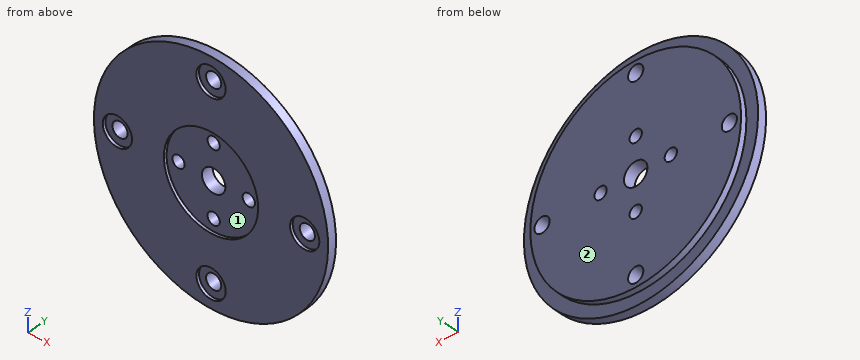
```python
from build123d import *

# Parameters (mm, degrees)
SKETCH_1_R               = 40
EXTRUDE_1_DEPTH          = 3
SKETCH_2_R               = 36
EXTRUDE_2_DEPTH          = 2
CUT_EXTRUDE_1_DEPTH      = 57.789083458
CUT_EXTRUDE_1_DEPTH_BACK = 57.789083458
SKETCH_3_R               = 2.1
SKETCH_3_R_2             = 4
SKETCH_4_R               = 16.1
CUT_EXTRUDE_2_DEPTH      = 1
SKETCH_5_R               = 2.6
CUT_EXTRUDE_3_DEPTH      = 57.789083458
SKETCH_6_R               = 5
CUT_EXTRUDE_4_DEPTH      = 1


with BuildPart() as part:
    # 草图1 → 凸台-拉伸1 (new body)
    with BuildSketch(Plane(origin=(0, 0, 0), x_dir=(1, 0, 0), z_dir=(0, 1, 0))):
        with Locations(Location((0, 0, 0), (0, 0, 270))):
            Circle(SKETCH_1_R)
    extrude(amount=EXTRUDE_1_DEPTH)

    # 草图2 → 凸台-拉伸2 (add)
    with BuildSketch(Plane(origin=(0, 3, 0), x_dir=(1, 0, 0), z_dir=(0, 1, 0))):
        with Locations(Location((0, 0, 0), (0, 0, 270))):
            Circle(SKETCH_2_R)
    extrude(amount=EXTRUDE_2_DEPTH)

    # 草图3 → 切除-拉伸1 (cut, two sides: drawn at the far end of the back side and taken through both)
    with BuildSketch(Plane.XZ.offset(-CUT_EXTRUDE_1_DEPTH_BACK)):
        with Locations(Location((-12, 0, 0), (0, 0, 270))):
            Circle(SKETCH_3_R)
        with Locations(Location((0, 12, 0), (0, 0, 270))):
            Circle(SKETCH_3_R)
        with Locations(Location((12, 0, 0), (0, 0, 270))):
            Circle(SKETCH_3_R)
        with Locations(Location((0, -12, 0), (0, 0, 270))):
            Circle(SKETCH_3_R)
        with Locations(Location((0, 0, 0), (0, 0, 270))):
            Circle(SKETCH_3_R_2)
    extrude(amount=CUT_EXTRUDE_1_DEPTH + CUT_EXTRUDE_1_DEPTH_BACK, mode=Mode.SUBTRACT)

    # 草图4 → 切除-拉伸2 (cut)
    with BuildSketch(Plane.XZ):
        with Locations(Location((0, 0, 0), (0, 0, 270))):
            Circle(SKETCH_4_R)
    extrude(amount=-CUT_EXTRUDE_2_DEPTH, mode=Mode.SUBTRACT)

    # 草图5 → 切除-拉伸3 (cut, through all)
    with BuildSketch(Plane.XZ):
        with Locations(Location((-32, 0, 0), (0, 0, 270))):
            Circle(SKETCH_5_R)
        with Locations(Location((0, 32, 0), (0, 0, 270))):
            Circle(SKETCH_5_R)
        with Locations(Location((32, 0, 0), (0, 0, 270))):
            Circle(SKETCH_5_R)
        with Locations(Location((0, -32, 0), (0, 0, 270))):
            Circle(SKETCH_5_R)
    extrude(amount=-CUT_EXTRUDE_3_DEPTH, mode=Mode.SUBTRACT)

    # 草图6 → 切除-拉伸4 (cut)
    with BuildSketch(Plane.XZ):
        with Locations(Location((0, -32, 0), (0, 0, 270))):
            Circle(SKETCH_6_R)
        with Locations(Location((32, 0, 0), (0, 0, 270))):
            Circle(SKETCH_6_R)
        with Locations(Location((0, 32, 0), (0, 0, 270))):
            Circle(SKETCH_6_R)
        with Locations(Location((-32, 0, 0), (0, 0, 270))):
            Circle(SKETCH_6_R)
    extrude(amount=-CUT_EXTRUDE_4_DEPTH, mode=Mode.SUBTRACT)


solid = part.part
```
Could you check a few things on this model? Use its own coordinates, in mm. Face numbers are marked on the shaded views. Round coordinates to 2 decimals unless told otherwise and drop trailing zeros. Loops run counter-clockwise (first coordinate to the right, second up) from the corner with the lowest first, then second, coordinate; pieces in that order, holes last. Notation, with made-up numbers: (29, -34.75) -> (55, -34.75) arc R24 ccw to (55, -21.75) -> close; hole circle Ø10 at (81, 68). An arc over 180 degrees is marked (long way). One line per question, with ' | ' between items.
(1) If we section it at A-A on y = 3.8: Count the separate pieces of the cut face and the enclosed holes in it, and give its area (3 significant figures).
Model answer:
separate pieces: 1 | enclosed holes: 9 | area: 3,880 mm^2
(2) For pin 1 Ø5 at (x, z) = (0, -30.5) entering from -Y; pin 2 Ø3 at (x, y) = (-8.5, 2) entering from +Z; pin 3 Ø2 at (y, z) = (2, -2.5) entering from -X, each with a flat end and sliding along its axis, tell me the tip position at first contact or that it passes through.
Model answer:
pin 1: stops at y = 1 | pin 2: stops at z = 39.38 | pin 3: stops at x = -39.97
(3) If we section it at C-C on x = -32: List the corners of the cut face in (y, z) for me.
Model answer:
outline: (0, -24) -> (3, -24) -> (3, -16.49) -> (5, -16.49) -> (5, -2.6) -> (1, -2.6) -> (1, -5) -> (0, -5) -> close; (0, 5) -> (1, 5) -> (1, 2.6) -> (5, 2.6) -> (5, 16.49) -> (3, 16.49) -> (3, 24) -> (0, 24) -> close
(4) If I drill on probe 1 along X at (y, z) = (3.15, 0); probe 2 along X at (y, z) = (2.9, 0); probe 3 along Y at (x, z) = (6.5, 9), over which ranges is the centre line in solid material (lowest first)?
Model answer:
probe 1: x = -36 to -34.6, -29.4 to -14.1, -9.9 to -4, 4 to 9.9, 14.1 to 29.4, 34.6 to 36 | probe 2: x = -40 to -34.6, -29.4 to -14.1, -9.9 to -4, 4 to 9.9, 14.1 to 29.4, 34.6 to 40 | probe 3: y = 1 to 5
(5) If we section it at B-B on z = -12: List the corners of the cut face in (x, y) for me, and give its area (3 significant figures).
Model answer:
outline: (-38.16, 0) -> (-10.73, 0) -> (-10.73, 1) -> (-2.1, 1) -> (-2.1, 5) -> (-33.94, 5) -> (-33.94, 3) -> (-38.16, 3) -> close; (2.1, 1) -> (10.73, 1) -> (10.73, 0) -> (38.16, 0) -> (38.16, 3) -> (33.94, 3) -> (33.94, 5) -> (2.1, 5) -> close | area: 326 mm^2
(6) Thinking about a two-plate mould opening in X: for the marked faces 1 and 2, which applies, released by +X, released by -X, zero draft, split by the parting line, or undercut?
Model answer:
face 1: undercut | face 2: zero draft
